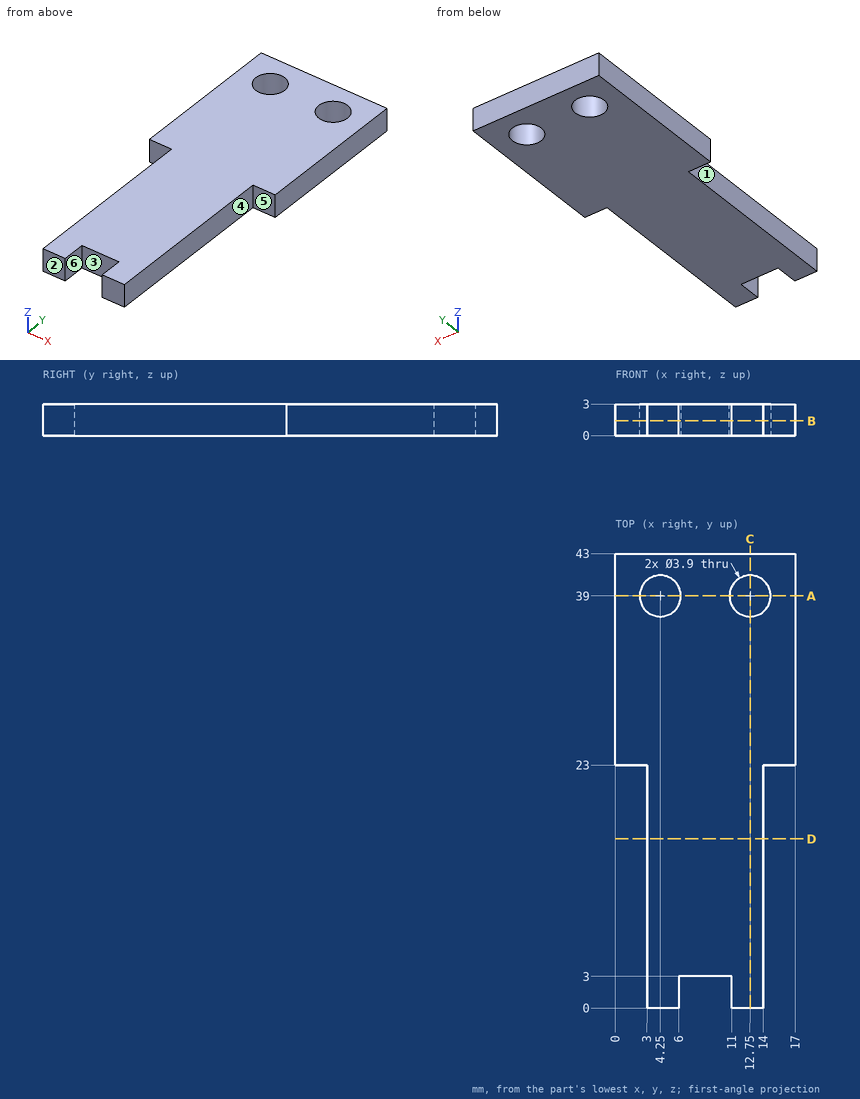
Verification items for this drawing (mm, ordinates from the low corner). A direction names the side the tool comes from. Round coordinates to 2 decimals unless told otherwise and drop trailing zeros. Order: outer loops, then holes, each group sorted by start corner. A loop starts at its lowest first (then second) coordinate and runs counter-clockwise, first axis right, second up. Notation, with made-up numbers: (13.25, 61.25) - (49.25, 61.25) arc R16 ccw to (49.25, 68.25) - close; hole circle Ø7 at (59.25, -4.5). An arc over 180 degrees is marked (long way). Use CSV: the item, a comma, the result in double quotes. Start each with the question number.
1) Section check C-C, the plane x = 12.75. Record the cut outline in (y, z).
2) Thickness scan on L1, parallel to Y at x = 4.25, z = 1.7; L2, parallel to Y at x = 15.25, z = 0.3; L3, parallel to X at y = 15, z = 0.6. Record the ranges inside material, lowest first.
3) Section check B-B, the plane z = 1.4. Record the cut outline in (x, y).
4) Go/stop test with a flat-tipped pin: P1, Ø1.5, axis at x = 15, z = 2, coming from the -Y side. Record where the tip stops, or that it passes through.
5) Section check D-D, the plane y = 16. Record the cut outline in (x, z).
6) Section check A-A, the plane y = 39. Record the cut outline in (x, z).
7) Mould release check, pull along X, two halves, no side actions. Record for the marked faces 4, 5 and 6: +X half, -X half, draft (parallel to the pull), parting line (faces both ways), or undercut.
8) Access from +Z, -Z, +X, -X, +Y, -Y to the whole of each face (thin tool, end or side, straight path). Record for the marked faces 1, 2 and 3.
Answers:
1,outline,"(0, 0) - (37.05, 0) - (37.05, 3) - (0, 3) - close; (40.95, 0) - (43, 0) - (43, 3) - (40.95, 3) - close"
2,L1,"y = 0 to 37.05, 40.95 to 43"
2,L2,"y = 23 to 43"
2,L3,"x = 3 to 14"
3,outline,"(0, 23) - (3, 23) - (3, 0) - (6, 0) - (6, 3) - (11, 3) - (11, 0) - (14, 0) - (14, 23) - (17, 23) - (17, 43) - (0, 43) - close; hole circle Ø3.9 at (4.25, 39); hole circle Ø3.9 at (12.75, 39)"
4,P1,"stops at y = 23"
5,outline,"(3, 0) - (14, 0) - (14, 3) - (3, 3) - close"
6,outline,"(0, 0) - (2.3, 0) - (2.3, 3) - (0, 3) - close; (6.2, 0) - (10.8, 0) - (10.8, 3) - (6.2, 3) - close; (14.7, 0) - (17, 0) - (17, 3) - (14.7, 3) - close"
7,face 4,"+X half"
7,face 5,"draft"
7,face 6,"undercut"
8,face 1,"+Z, -Z, -X, -Y"
8,face 2,"+Z, -Z, +X, -X, -Y"
8,face 3,"+Z, -Z, -Y"
